```python
from build123d import *

# Parameters (mm, degrees)
F0_W     = 19.05
F0_H     = 19.05
F1_DEPTH = 19.05
F3_DEPTH = 25.4
F4_W     = 1.27
F4_H     = 6.35
F5_DEPTH = 2.54
F6_W     = 1.27
F6_H     = 6.35
F7_DEPTH = 2.54


with BuildPart() as f1:
    # F0 (on Top) → F1 (new body)
    with BuildSketch(Plane.XY):
        with Locations((-43.75411, 52.740463)):
            Rectangle(F0_W, F0_H)
    extrude(amount=F1_DEPTH)

    # F2 (on face) → F3 (cut)
    with BuildSketch(Plane.XY.offset(19.05)):
        with BuildLine():
            Line((-34.22911, 62.265463), (-40.196911, 62.265463))
            ThreePointArc((-40.196911, 62.265463), (-37.927985, 58.014519), (-34.22911, 54.926336))
            Line((-34.22911, 54.926336), (-34.22911, 62.265463))
        make_face()
    extrude(amount=-F3_DEPTH, mode=Mode.SUBTRACT)

    # F4 (on face) → F5 (join)
    with BuildSketch(Plane.YZ.offset(-34.22911)):
        with Locations((54.291336, 9.525)):
            Rectangle(F4_W, F4_H)
    extrude(amount=F5_DEPTH)

    # F6 (on face) → F7 (join)
    with BuildSketch(Plane(origin=(0, 62.265463, 0), x_dir=(-1, 0, 0), z_dir=(0, 1, 0))):
        with Locations((40.831911, 9.525)):
            Rectangle(F6_W, F6_H)
    extrude(amount=F7_DEPTH)


solid = f1.part
```
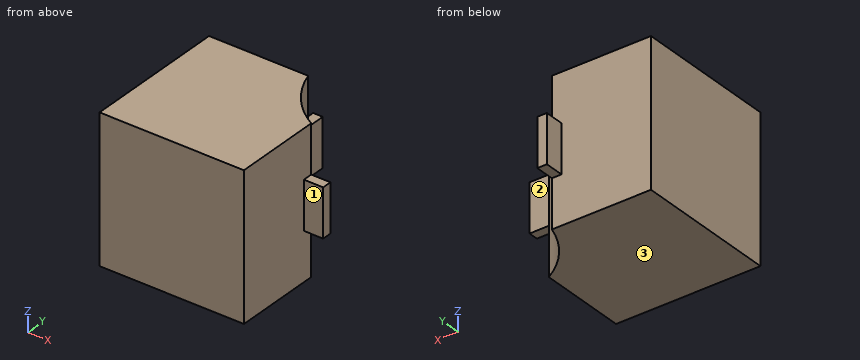
Source: CAD feature listing. Evaluate the final solid. Frame: model axes, mm. Face numbers are marked on the shaded views. A direction names the side the tool comes from. Give positions to 0.01 mm unless a question says otherwise; leave off trailing zeros. Loops run counter-clockwise (first coordinate to the right, second up) from the corner with the lowest first, then second, coordinate; pieces in that order, holes last. Notation, with made-up numbers: (86.25, 66.5) -> (114.25, 66.5) arc R31 ccw to (114.25, 97.5) -> close; hole circle Ø3 at (-3.75, 55). An arc over 180 degrees is marked (long way). Put each result on its own line as item: value. Start each with the question number.
1) Cut plane B-B (z = 8.75). Return loops of the section in (x, y), then the cut area to 3 significant figures.
2) Cut plane C-C (x = -47.25). Return loops of the section in (y, z), then the cut area to 3 significant figures.
3) Contact query for flat-ended pins moving along their axis: P1, Ø10, axis at x = -35, y = 60.5, coming from the -Z side; P2, Ø1, axis at x = -33, y = 54, coming from the +Z side; P3, Ø1.3, axis at x = -33, z = 10, coming from the -Y side; P4, Ø1.4, axis at x = -40.5, y = 63.5, coming from the -Z side. Output: stop coordinate, or through.
4) Cut plane A-A (y = 54). Return loops of the section in (x, z), then the cut area to 3 significant figures.
5) Cut plane D-D (z = 16.25). Return loops of the section in (x, y), then the cut area to 3 significant figures.
6) Material intervals for probe 1 along Y at (x, z) = (-49.75, 8); probe 2 along X at (y, z) = (50, 6.75); probe 3 along Y at (x, z) = (-33.75, 11.5), sorted ascending.
7) Reachability of the marked faces 1, 2 and 3 from +Z, -Z, +X, -X, +Y, -Y: full face, straight path, thin tool, end or side. Return the list, or none.
Results are:
1. outline: (-53.28, 43.22) -> (-34.23, 43.22) -> (-34.23, 53.66) -> (-31.69, 53.66) -> (-31.69, 54.93) -> (-34.23, 54.93) arc R12.6 cw to (-40.2, 62.27) -> (-40.2, 64.81) -> (-41.47, 64.81) -> (-41.47, 62.27) -> (-53.28, 62.27) -> close
1. area: 342 mm2
2. outline: (43.22, 0) -> (62.27, 0) -> (62.27, 19.05) -> (43.22, 19.05) -> close
2. area: 363 mm2
3. P1: stops at z = 0
3. P2: stops at z = 12.7
3. P3: stops at y = 53.66
3. P4: stops at z = 6.35
4. outline: (-53.28, 0) -> (-34.23, 0) -> (-34.23, 6.35) -> (-31.69, 6.35) -> (-31.69, 12.7) -> (-34.23, 12.7) -> (-34.23, 19.05) -> (-53.28, 19.05) -> close
4. area: 379 mm2
5. outline: (-53.28, 43.22) -> (-34.23, 43.22) -> (-34.23, 54.93) arc R12.6 cw to (-40.2, 62.27) -> (-53.28, 62.27) -> close
5. area: 335 mm2
6. probe 1: y = 43.22 to 62.27
6. probe 2: x = -53.28 to -34.23
6. probe 3: y = 53.66 to 54.93
7. face 1: +Z, -Z, +X, -Y
7. face 2: +Z, -Z, +X, +Y
7. face 3: -Z, +X, -X, +Y, -Y
